Geometry: final body of the model. Coordinates: model frame, mm. A direction names the side the tool comes from. Round coordinates to 2 decimals unless told otherwise and drop trailing zeros. Order: outer loops, then holes, each group sorted by start corner. A loop starts at its lowest first (then second) coordinate and runs counter-clockwise, first axis right, second up. Notation, with made-up numbers: (79, 5) - (135, 5) arc R28 ccw to (135, 41) - close; hole circle Ø4 at (67.25, 55.5). An arc over 180 degrees is marked (long way). Put each result on its own line as item: value. Start each with the question number.
(1) Section D-D (z = -1.5). Output: boundary loops of the cut face in (x, y), and give its area (3 significant figures).
(2) Material intervals for L1, parallel to Y at x = 0, z = 0.75; L2, parallel to Y at x = -2, z = 2.5; L3, parallel to Y at x = 0.25, z = 2.75, sorted ascending. Write a range as [from, to].
(3) Access query for faces 5 (the face through (3.535, 26.716, 2.493)), 6 (the face through (1.51, 32.36, 2.01)), 7 (the face through (-3.535, 26.716, -2.493)), 8 (the face through (3.48, 26.62, -2.49)). Directions: +Z, -Z, +X, -X, +Y, -Y. A direction counts if a zero-diameter tool reaches every point of the face in a straight line with its end or side. Return the directions, or none.
(4) Section C-C (z = 0.25). Output: boundary loops of the cut face in (x, y), and give its area (3 significant figures).
(5) Pin query (flat end, axial travel): P1, Ø3, axis at x = 3, y = 13.5, coming from the -Z side; P2, Ø3.5, axis at x = 0, y = 30, coming from the +Z side; P3, Ø3, axis at y = 28, z = 1.5, coming from the -X side. Return the tip coordinate at first contact, or that it passes through.
(6) Section A-A (x = 0). Count the separate pieces of the cut face and the enclosed holes in it, and give its area (3 significant figures).
(7) Pull-direction query (Y, two-part tool) for faces 1 (the face through (4.42, 2.74, -0.03)), 2 (the face through (4.5, 32.6, 0)), 3 (the face through (0.042, -4.703, 2.493)), 4 (the face through (0, 14, 3)); classes: released by +Y, released by -Y, zero draft, split by the parting line, or undercut.
(8) Section B-B (y = 8). Output: boundary loops of the cut face in (x, z).
Autodesk Inventor part; units mm, degrees
ref_plane "YZ Plane" through (0, 0, 0) normal (1, 0, 0) x (0, 1, 0)
ref_plane "XZ Plane" through (0, 0, 0) normal (0, 1, 0) x (-1, 0, 0)
ref_plane "XY Plane" through (0, 0, 0) normal (0, 0, 1) x (1, 0, 0)
sketch "Sketch1" plane through (0, 0, 0) normal (0, 0, 1) x (1, 0, 0)
  circle A0 centre (0, 0) radius 1.55
  circle A1 centre (0, 0) radius 3
  line L0 (0, 0) -> (0, 30)
  circle A2 centre (0, 30) radius 1.55
  circle A3 centre (0, 30) radius 3
  line L1 (3, 0) -> (3, 30)
  line L2 (-3, 0) -> (-3, 30)
  line L3 (6, 30) -> (3, 24.8038)
  line L4 (3, 24.8038) -> (-3, 24.8038)
  line L5 (-3, 24.8038) -> (-6, 30)
  line L6 (-6, 30) -> (-3, 35.1962)
  line L7 (-3, 35.1962) -> (3, 35.1962)
  line L8 (3, 35.1962) -> (6, 30)
  line L9 (6, 0) -> (3, -5.1962)
  line L10 (3, -5.1962) -> (-3, -5.1962)
  line L11 (-3, -5.1962) -> (-6, 0)
  line L12 (-6, 0) -> (-3, 5.1962)
  line L13 (-3, 5.1962) -> (3, 5.1962)
  line L14 (3, 5.1962) -> (6, 0)
  point P0 (3, 24.8038)
  point P1 (-3, 24.8038)
  dimension "d0" = 3.1
  dimension "d1" = 6
  dimension "d2" = 30
  dimension "d3" = 3.1
  dimension "d4" = 6
  dimension "d5" = 30
  dimension "d6" = 3
  dimension "d7" = 6
  dimension "d8" = 6
extrude "Extrusion1" add sketch "Sketch1" along normal blind 3
sketch "Sketch2" plane through (0, 0, 3) normal (0, 0, 1) x (1, 0, 0)
  circle A0 centre (0, 0) radius 2.8
  line L0 (3, 5.1962) -> (3, 24.8038)
  line L1 (3, 24.8038) -> (6, 30)
  line L2 (6, 30) -> (3, 35.1962)
  line L3 (3, 35.1962) -> (-3, 35.1962)
  line L4 (-3, 35.1962) -> (-6, 30)
  line L5 (-6, 30) -> (-3, 24.8038)
  line L6 (-3, 24.8038) -> (-3, 5.1962)
  line L7 (-3, 5.1962) -> (-6, 0)
  line L8 (-6, 0) -> (-3, -5.1962)
  line L9 (-3, -5.1962) -> (3, -5.1962)
  line L10 (3, -5.1962) -> (6, 0)
  line L11 (6, 0) -> (3, 5.1962)
  circle A1 centre (0, 30) radius 1.55
  circle A2 centre (0, 0) radius 1.55
  circle A3 centre (0, 30) radius 2.8
  dimension "d11" = 5.6
  dimension "d12" = 5.6
extrude "Extrusion2" cut sketch "Sketch2" against normal blind 2 contours A0 | A3
chamfer "Chamfer1" distance 2 angle 45 2 edges at (-3, 15, 3) (3, 15, 3)
chamfer "Chamfer2" distance 1 angle 45 10 edges at (-4.5, 2.5981, 3) (-4.5, -2.5981, 3) (0, -5.1962, 3) (4.5, -2.5981, 3) (4.5, 2.5981, 3) (4.5, 27.4019, 3) (-4.5, 27.4019, 3) (4.5, 32.5981, 3) (0, 35.1962, 3) (-4.5, 32.5981, 3)
mirror "Mirror1" about plane through (0, 15, 0) normal (0, 0, -1)
equation "\"d0\" = d3"
equation "\"d1\" = d4"
equation "\"d5\" = d2"
equation "\"d12\" = d11"
properties part number "Tibia Joint"
Checks:
1. outline: (-6, 0) - (-3, -5.2) - (3, -5.2) - (6, 0) - (2.5, 6.06) - (2.5, 23.94) - (6, 30) - (3, 35.2) - (-3, 35.2) - (-6, 30) - (-2.5, 23.94) - (-2.5, 6.06) - close; hole circle Ø5.6 at (0, 0); hole circle Ø5.6 at (0, 30)
1. area: 237 mm²
2. L1: y = [-5.2, -1.55], [1.55, 28.45], [31.55, 35.2]
2. L2: y = [-4.7, -1.96], [1.96, 5.93], [24.07, 28.04], [31.96, 34.7]
2. L3: y = [-4.45, -2.79], [2.79, 27.21], [32.79, 34.45]
3. face 5: +Z, +X
3. face 6: +Z
3. face 7: -Z, -X
3. face 8: -Z, +X
4. outline: (-6, 0) - (-3, -5.2) - (3, -5.2) - (6, 0) - (3, 5.2) - (3, 24.8) - (6, 30) - (3, 35.2) - (-3, 35.2) - (-6, 30) - (-3, 24.8) - (-3, 5.2) - close; hole circle Ø3.1 at (0, 0); hole circle Ø3.1 at (0, 30)
4. area: 290 mm²
5. P1: stops at z = -2.5
5. P2: stops at z = 1
5. P3: stops at x = -5.71
6. separate pieces: 3
6. enclosed holes: 0
6. area: 183 mm²
7. face 1: undercut
7. face 2: released by +Y
7. face 3: released by -Y
7. face 4: zero draft
8. outline: (-3, -1) - (-1, -3) - (1, -3) - (3, -1) - (3, 1) - (1, 3) - (-1, 3) - (-3, 1) - close
